Check sheet for the drawn part. Datum: minimum x, y, z corner. Units: mm. A direction names the side the tool comes from. Round coordinates to 2 decimals unless told otherwise and drop trailing zeros. Loops run counter-clockwise (first coordinate to the right, second up) from the corner with the lowest first, then second, coordinate; pieces in that order, holes last.
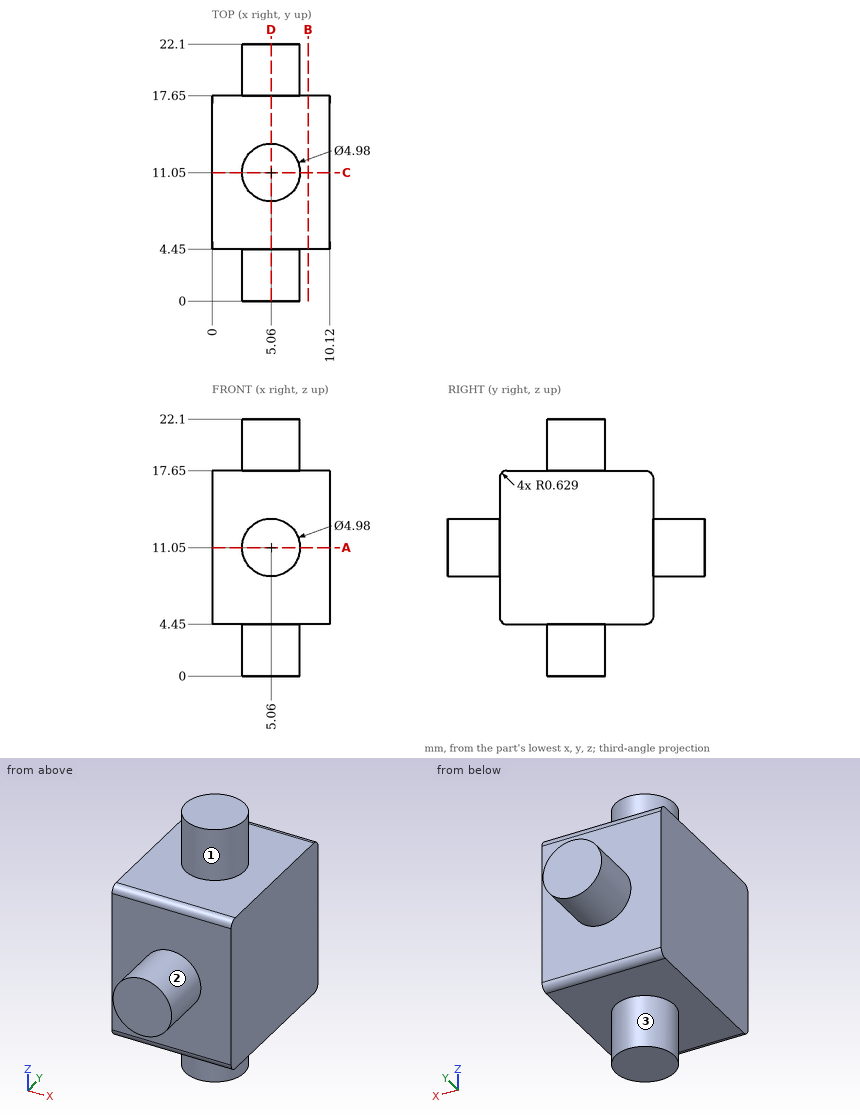
1) Gauge pin test, flat ends, axial feed: pin 1 (6 mm diameter, centred on x = 2, z = 18.5, fed in from -Y); pin 2 (4 mm diameter, centred on x = 7.5, z = 4, fed in from +Y); pin 3 (2 mm diameter, centred on x = 9, y = 4, fed in from +Z) (1 decimal); pin 4 (2 mm diameter, centred on x = 1.5, z = 2.5, fed in from -Y) (3 decimals). Record the tip position at first contact, or that the pin passes through.
Report:
pin 1: stops at y = 4.45
pin 2: stops at y = 17.65
pin 3: stops at z = 17.6
pin 4: passes through
2) Sectioned sample at B-B, the plane x = 8.25. Record the cut outline in (y, z).
Report:
outline: (4.45, 5.08) arc R0.63 ccw to (5.08, 4.45) - (17.02, 4.45) arc R0.63 ccw to (17.65, 5.08) - (17.65, 17.02) arc R0.63 ccw to (17.02, 17.65) - (5.08, 17.65) arc R0.63 ccw to (4.45, 17.02) - close
3) Sectioned sample at A-A, the plane z = 11.05. Record the cut outline in (x, y).
Report:
outline: (0, 4.45) - (2.57, 4.45) - (2.57, 0) - (7.55, 0) - (7.55, 4.45) - (10.12, 4.45) - (10.12, 17.65) - (7.55, 17.65) - (7.55, 22.1) - (2.57, 22.1) - (2.57, 17.65) - (0, 17.65) - close
4) Scan lines: line 1 along Y through (x, z) = (2.75, 7); line 2 along Y through (x, z) = (3.5, 1.5). Record each from-to range of solid material in increasing order.
Report:
line 1: y = 4.45 to 17.65
line 2: y = 9.11 to 12.99
5) Sectioned sample at D-D, the plane x = 5.06. Record the cut outline in (y, z).
Report:
outline: (0, 8.56) - (4.45, 8.56) - (4.45, 5.08) arc R0.63 ccw to (5.08, 4.45) - (8.56, 4.45) - (8.56, 0) - (13.54, 0) - (13.54, 4.45) - (17.02, 4.45) arc R0.63 ccw to (17.65, 5.08) - (17.65, 8.56) - (22.1, 8.56) - (22.1, 13.54) - (17.65, 13.54) - (17.65, 17.02) arc R0.63 ccw to (17.02, 17.65) - (13.54, 17.65) - (13.54, 22.1) - (8.56, 22.1) - (8.56, 17.65) - (5.08, 17.65) arc R0.63 ccw to (4.45, 17.02) - (4.45, 13.54) - (0, 13.54) - close
6) Access from +Z, -Z, +X, -X, +Y, -Y to the whole of each face (thin tool, end or side, straight path). Record for the marked faces 1, 2 and 3.
Report:
face 1: +Z
face 2: -Y
face 3: -Z
